Part model, mm, in its own coordinate system. Face numbers are marked on the shaded views. A direction names the side the tool comes from. Give positions to 0.01 mm unless a question says otherwise; leave off trailing zeros. Loops run counter-clockwise (first coordinate to the right, second up) from the corner with the lowest first, then second, coordinate; pieces in that order, holes last. Notation, with made-up numbers: M 58,17.5 L 111,17.5 A4 cw 111,24.5 Z; hole C 30,-31 d7. An arc over 180 degrees is marked long. Answer in a Markdown table with one row per item.
from build123d import *

# Parameters (mm, degrees)
BOSS_EXTRUDE1_DEPTH = 5


with BuildPart() as part:
    # Sketch1 → Boss-Extrude1 (new, symmetric)
    with BuildSketch(Plane(origin=(0, 0, 0), x_dir=(1, 0, 0), z_dir=(0, 1, 0))):
        with BuildLine():
            Line((1.5, 0), (-1.5, 0))
            ThreePointArc((-1.5, 0), (-2.96457943, 3.057716073), (-0.642857143, 5.528389282))
            ThreePointArc((-0.642857143, 5.528389282), (-0.261614488, 6.123917651), (-0.857142857, 6.505160306))
            ThreePointArc((-0.857142857, 6.505160306), (-3.972144627, 3.069316131), (-1.747526131, -1))
            Line((-1.747526131, -1), (1.747526131, -1))
            ThreePointArc((1.747526131, -1), (3.972144627, 3.069316131), (0.857142857, 6.505160306))
            ThreePointArc((0.857142857, 6.505160306), (0.261614488, 6.123917651), (0.642857143, 5.528389282))
            ThreePointArc((0.642857143, 5.528389282), (2.96457943, 3.057716073), (1.5, 0))
        make_face()
    extrude(amount=BOSS_EXTRUDE1_DEPTH, both=True)


solid = part.part
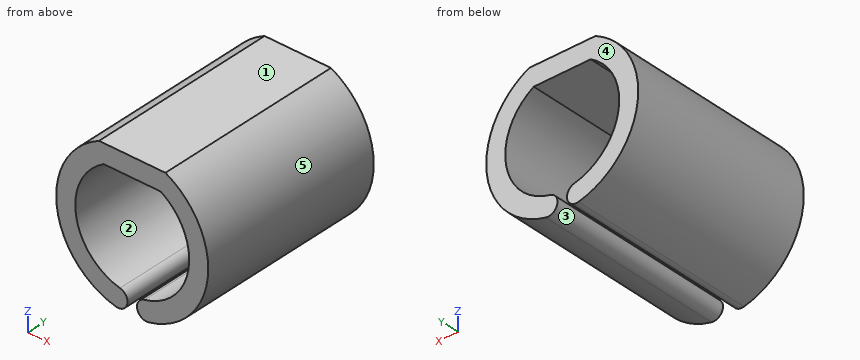
(1) Drill centre lines: line 1 along Z through (x, y) = (-1.75, -0.5); line 2 along X through (y, z) = (0.75, -6); line 3 along Z through (x, y) = (-2.75, -1.75). Where is each one in solid material? Low to high.
Recorded:
| item | result |
|---|---|
| line 1 | z = -6.19 to -5.03, -0.16 to 1 |
| line 2 | x = -2.1 to -0.25, 0.25 to 2.1 |
| line 3 | z = -5.5 to -3.8, -1.4 to 0.31 |
(2) Saw through at A-A (z = -3.75). Write the cut outline in (x, y).
Recorded:
| item | result |
|---|---|
| outline | M -3.83,-5 L -2.77,-5 L -2.77,5 L -3.83,5 Z; M 2.77,-5 L 3.83,-5 L 3.83,5 L 2.77,5 Z |
(3) Saw through at D-D (z = 0.25). Write the cut outline in (x, y).
Recorded:
| item | result |
|---|---|
| outline | M -2.81,-5 L 2.81,-5 L 2.81,5 L -2.81,5 Z |
(4) Pull direction X, two halves, no side cores. Call the marked faces 3, 4 and 5: +X half, -X half, draft (parallel to the pull), parting line (faces both ways), or undercut.
Recorded:
| item | result |
|---|---|
| face 3 | undercut |
| face 4 | draft |
| face 5 | +X half |
(5) Pin check, flat tips, straight feed: pin 1 Ø1.5 at (y, z) = (-1, -0.5) entering from +X; pin 2 Ø1 at (x, y) = (2.5, -1) entering from +Z. Stop position of each tip, or through.
Recorded:
| item | result |
|---|---|
| pin 1 | stops at x = 3.77 |
| pin 2 | stops at z = 0.87 |
(6) Which spindle directions (+Z, -Z, +X, -X, +Y, -Y) get a long thin tool onto all of the face, cutting with end or side? Do the marked faces 1 and 2. Say none if no direction does.
Recorded:
| item | result |
|---|---|
| face 1 | +Z, +X, -X, +Y, -Y |
| face 2 | +Y, -Y |
(7) Saw through at C-C (y = 3). Write the cut outline in (x, z).
Recorded:
| item | result |
|---|---|
| outline | M -1.75,1 A4 ccw -0.86,-6.51 A0.5 ccw -0.64,-5.53 A3 cw -1.5,0 L 1.5,0 A3 cw 0.64,-5.53 A0.5 ccw 0.86,-6.51 A4 ccw 1.75,1 Z |
(8) Saw through at B-B (x = 2.75). Write the cut outline in (y, z).
Recorded:
| item | result |
|---|---|
| outline | M -5,-5.5 L 5,-5.5 L 5,-3.8 L -5,-3.8 Z; M -5,-1.4 L 5,-1.4 L 5,0.31 L -5,0.31 Z |
